Geometry check sheet. Reference: drawing and pictorial views, mm from the part's lowest x, y, z. Round coordinates to 2 decimals unless told otherwise and drop trailing zeros. Write each loop counter-clockwise with the first axis right and the second up, starting at its lowest first coordinate (ties: lowest second). Pieces come first, ordered by that corner, then holes. Notation, with made-up numbers: (88, 32) -> (145, 32) arc R13 cw to (145, 53) -> close; hole circle Ø7 at (55, 33). An arc over 180 degrees is marked (long way). Answer as a JSON object with one key per item and string values. Group by question number.
(1) Sectioned sample at A-A on x = 30.5. Record the cut outline in (y, z).
(2) Sectioned sample at C-C on z = 7.75. Record the cut outline in (x, y) (1 decimal), and give its area (3 significant figures).
(3) Gauge pin test, flat ends, axial feed: pin 1 Ø4.5 at (x, y) = (23.15, 9.89) entering from +Z; pin 2 Ø4 at (y, z) = (14, 3.5) entering from -X; pin 3 Ø5 at (y, z) = (27.5, 3.5) entering from +X (1 decimal); pin 4 Ø3 at (y, z) = (39.5, 5.5) entering from -X. Record the tip position at first contact, or that the pin passes through.
(4) Sectioned sample at B-B on y = 32.5. Record the cut outline in (x, z).
(5) Sectioned sample at D-D on y = 24.5. Record the cut outline in (x, z) (1 decimal).
(6) Scan lines: L1, parallel to X at y = 10.5, z = 4 (1 decimal); L2, parallel to Y at x = 39, z = 2 (1 decimal); L3, parallel to X at y = 8.5, z = 2.5 (1 decimal). Record each from-to range of solid material in increasing order. Write a range as from..to.
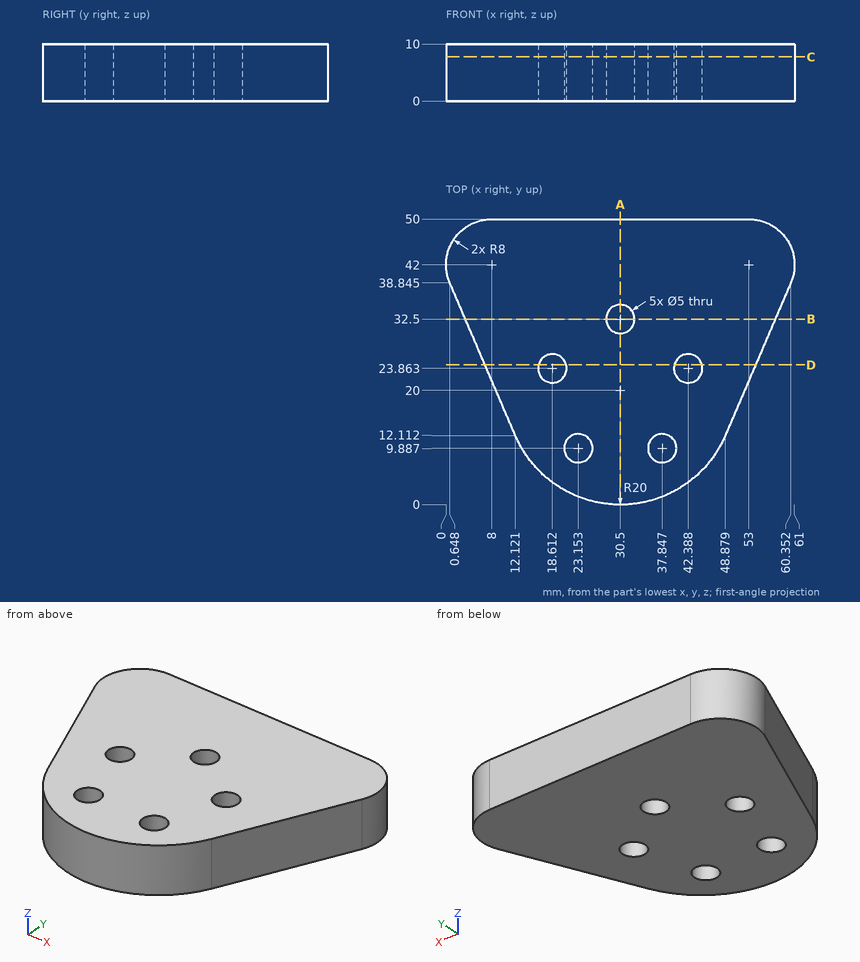
Computed values:
{
 "1": {"outline": "(0, 0) -> (30, 0) -> (30, 10) -> (0, 10) -> close; (35, 0) -> (50, 0) -> (50, 10) -> (35, 10) -> close"},
 "2": {"outline": "(0.6, 38.8) -> (12.1, 12.1) arc R20 ccw to (48.9, 12.1) -> (60.4, 38.8) arc R8 ccw to (53, 50) -> (8, 50) arc R8 ccw to start; hole circle Ø5 at (18.6, 23.9); hole circle Ø5 at (23.2, 9.9); hole circle Ø5 at (30.5, 32.5); hole circle Ø5 at (37.8, 9.9); hole circle Ø5 at (42.4, 23.9)", "area": "2,160 mm2"},
 "3": {"pin 1": "through", "pin 2": "x = 10.45", "pin 3": "x = 56.6", "pin 4": "x = 0.06"},
 "4": {"outline": "(3.37, 0) -> (28, 0) -> (28, 10) -> (3.37, 10) -> close; (33, 0) -> (57.63, 0) -> (57.63, 10) -> (33, 10) -> close"},
 "5": {"outline": "(6.8, 0) -> (16.2, 0) -> (16.2, 10) -> (6.8, 10) -> close; (21, 0) -> (40, 0) -> (40, 10) -> (21, 10) -> close; (44.8, 0) -> (54.2, 0) -> (54.2, 10) -> (44.8, 10) -> close"},
 "6": {"L1": "12.9..20.7, 25.6..35.4, 40.3..48.1", "L2": "1.9..7.7, 12.1..50", "L3": "14.1..21.1, 25.2..35.8, 39.9..46.9"}
}
